```python
from build123d import *


with BuildPart() as part:
    # Sketch1 → Revolve1 (revolve)
    with BuildSketch(Plane(origin=(0, 0, 0), x_dir=(-1, 0, 0), z_dir=(0, 0, -1))):
        with BuildLine():
            Line((-9.4, 4.2), (-9.5, 4.2))
            Line((-9.5, 4.2), (-9.5, 3))
            Line((-9.5, 3), (9.5, 3))
            Line((9.5, 3), (9.5, 4.2))
            Line((9.5, 4.2), (9.4, 4.2))
            Line((9.4, 4.2), (9.4, 4.3))
            Line((9.4, 4.3), (9.5, 4.3))
            Line((9.5, 4.3), (9.5, 4.9))
            ThreePointArc((9.5, 4.9), (9.470710678, 4.970710678), (9.4, 5))
            Line((9.4, 5), (6.8, 5))
            Line((6.8, 5), (6.8, 4.8))
            Line((6.8, 4.8), (5.65, 4.8))
            Line((5.65, 4.8), (5.65, 5))
            Line((5.65, 5), (-5.65, 5))
            Line((-5.65, 5), (-5.65, 4.8))
            Line((-5.65, 4.8), (-6.8, 4.8))
            Line((-6.8, 4.8), (-6.8, 5))
            Line((-6.8, 5), (-9.4, 5))
            ThreePointArc((-9.4, 5), (-9.470710678, 4.970710678), (-9.5, 4.9))
            Line((-9.5, 4.9), (-9.5, 4.3))
            Line((-9.5, 4.3), (-9.4, 4.3))
            Line((-9.4, 4.3), (-9.4, 4.2))
        make_face()
    revolve(axis=Axis((9.5, 0, 0), (-1, 0, 0)))


solid = part.part
```
Here's how the part is built. I have some questions about the finished solid (model axes, mm). Round coordinates to 2 decimals unless told otherwise and drop trailing zeros. Order: outer loops, then holes, each group sorted by start corner. A loop starts at its lowest first (then second) coordinate and runs counter-clockwise, first axis right, second up. Notation, with made-up numbers: M -3,44 L 33,44 A11 ccw 33,51 Z; hole C -33,22 d11. An arc over 180 degrees is marked long. Answer as CSV lines item,"result".
Item 1: For pin 1 (5.5 mm diameter, centred on y = 0, z = 0, fed in from +X); pin 2 (1.5 mm diameter, centred on x = -3, z = -1, fed in from -Y), each with a flat end and sliding along its axis, tell me the tip position at first contact or that it passes through.
From the geometry:
pin 1,"through"
pin 2,"y = -4.99"
Item 2: Imagine slicing it at A-A on x = 1.5. List the corners of the cut face in (y, z) for me, and give its area (3 significant figures).
From the geometry:
outline,"C 0,0 d10; hole C 0,0 d6"
area,"50.3 mm2"
Item 3: We'd pull the mould along X, two halves only. Please class faces 1 (the flat face through (9.5, 2, 4)), 2 (the flat face through (-9.5, 1, -3)), 3 (the cylindrical face through (-6.22, 2.58, -4.05)): +X half, -X half, draft (parallel to the pull), parting line (faces both ways), or undercut.
From the geometry:
face 1,"+X half"
face 2,"-X half"
face 3,"undercut"
Item 4: Please list where these lines run through material, in increasing order: L1, parallel to X at y = 1.75, z = -4.5; L2, parallel to Z at x = 2, y = 0. Write a range as [from, to].
From the geometry:
L1,"[-9.5, -6.8], [-5.65, 5.65], [6.8, 9.5]"
L2,"[-5, -3], [3, 5]"
